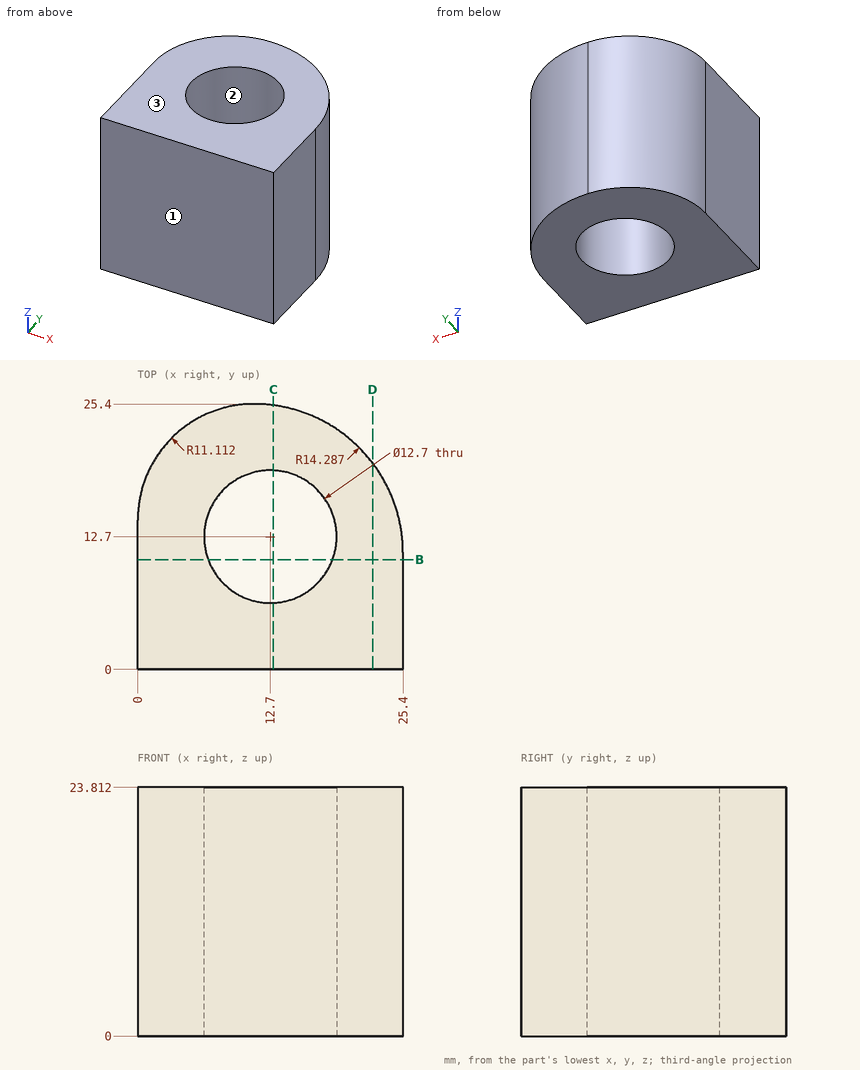
Design review of the part shown in the three views and the two pictorial views. Dimensions are in mm from the part's minimum x, y and z. Round coordinates to 2 decimals unless told otherwise and drop trailing zeros. Write each loop counter-clockwise with the first axis right and the second up, starting at its lowest first coordinate (ties: lowest second). Pieces come first, ordered by that corner, then holes.
Item 1: We need section D-D on x = 22.5. Write out the cut boundary in (y, z), and give its area (3 significant figures).
Item 2: Clearance check with flat-ended pins moving along their axes: pin 1 Ø3 at (x, z) = (15, 19) entering from +Y; pin 2 Ø12 at (x, z) = (20.5, 4.5) entering from +Y; pin 3 Ø3 at (y, z) = (13, 4) entering from +X (1 decimal). State where each tip first meets the part, or that it passes through.
Item 3: For probe 1 along X at (y, z) = (8.25, 18); probe 2 along X at (y, z) = (9.75, 14) (1 decimal); probe 3 along Y at (x, z) = (17, 18) (1 decimal), list the stretches that pass through material, from the lowest coordinate up.
Item 4: We need section B-B on y = 10.5. Write out the cut boundary in (x, z), and give its area (3 significant figures).
Item 5: The part is to be moulded in two halves that separate along Y. For the marked faces 1, 2 and 3, say which applies: +Y half, -Y half, draft (parallel to the pull), parting line (faces both ways), or undercut.
Item 6: We need section C-C on x = 13. Write out the cut boundary in (y, z) (1 decimal).
Returned:
1. outline: (0, 0) - (19.74, 0) - (19.74, 23.81) - (0, 23.81) - close
1. area: 470 mm2
2. pin 1: stops at y = 25.2
2. pin 2: stops at y = 24.99
2. pin 3: stops at x = 25.4
3. probe 1: x = 0 to 8.17, 17.23 to 25.4
3. probe 2: x = 0 to 7.1, 18.3 to 25.4
3. probe 3: y = 0 to 8, 17.4 to 24.1
4. outline: (0, 0) - (6.74, 0) - (6.74, 23.81) - (0, 23.81) - close; (18.66, 0) - (25.4, 0) - (25.4, 23.81) - (18.66, 23.81) - close
4. area: 321 mm2
5. face 1: -Y half
5. face 2: undercut
5. face 3: draft
6. outline: (0, 0) - (6.4, 0) - (6.4, 23.8) - (0, 23.8) - close; (19, 0) - (25.3, 0) - (25.3, 23.8) - (19, 23.8) - close
